Check sheet for the drawn part. Datum: minimum x, y, z corner. Units: mm. Round coordinates to 2 decimals unless told otherwise and drop trailing zeros. Order: outer loops, then holes, each group sorted by start corner. A loop starts at its lowest first (then second) coordinate and runs counter-clockwise, first axis right, second up. Notation, with made-up numbers: (48.5, 69) -> (77.5, 69) arc R16 cw to (77.5, 99) -> close; hole circle Ø10 at (-19, 65.5). An arc over 180 degrees is marked (long way). Use CSV: the item, a comma, the result in double quotes.
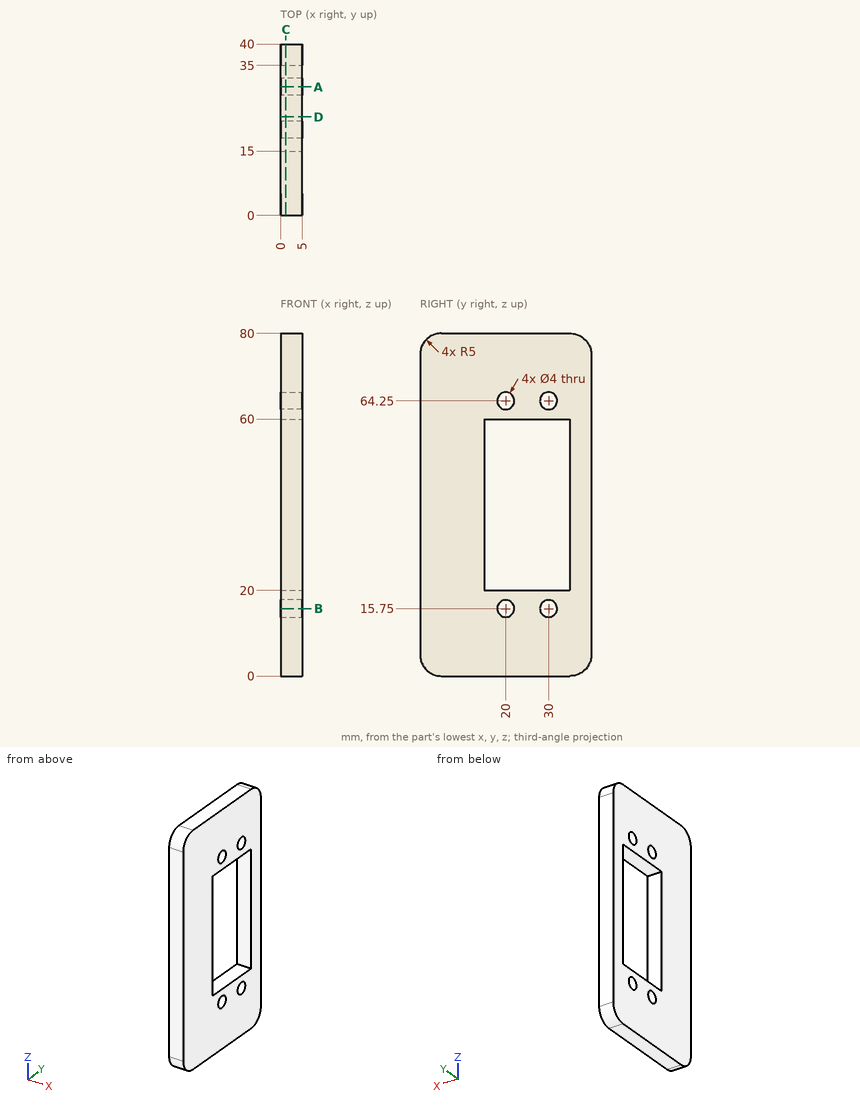
Q1. Sectioned sample at D-D, the plane y = 23. Enter the section's corners in (x, z).
Result sheet:
outline,"(0, 0) -> (5, 0) -> (5, 20) -> (0, 20) -> close; (0, 60) -> (5, 60) -> (5, 80) -> (0, 80) -> close"
Q2. Sectioned sample at C-C, the plane x = 1.2. Enter the section's corners in (y, z), then the cut area to 3 significant figures.
Result sheet:
outline,"(0, 5) arc R5 ccw to (5, 0) -> (35, 0) arc R5 ccw to (40, 5) -> (40, 75) arc R5 ccw to (35, 80) -> (5, 80) arc R5 ccw to (0, 75) -> close; hole (15, 20) -> (35, 20) -> (35, 60) -> (15, 60) -> close; hole circle Ø4 at (20, 15.75); hole circle Ø4 at (20, 64.25); hole circle Ø4 at (30, 15.75); hole circle Ø4 at (30, 64.25)"
area,"2,330 mm^2"
Q3. Go/stop test with a flat-tipped pin: pin 1 (3.5 mm diameter, centred on y = 20, z = 15.75, fed in from +X). Record where the tip stops, or that it passes through.
Result sheet:
pin 1,"passes through"
Q4. Scan lines: L1, parallel to Y at x = 1.35, z = 64.25; L2, parallel to Y at x = 1.6, z = 52.5; L3, parallel to Z at x = 2.35, y = 17. Record each from-to range of solid material in increasing order.
Result sheet:
L1,"y = 0 to 18, 22 to 28, 32 to 40"
L2,"y = 0 to 15, 35 to 40"
L3,"z = 0 to 20, 60 to 80"
Q5. Sectioned sample at A-A, the plane y = 30. Enter the section's corners in (x, z).
Result sheet:
outline,"(0, 0) -> (5, 0) -> (5, 13.75) -> (0, 13.75) -> close; (0, 17.75) -> (5, 17.75) -> (5, 20) -> (0, 20) -> close; (0, 60) -> (5, 60) -> (5, 62.25) -> (0, 62.25) -> close; (0, 66.25) -> (5, 66.25) -> (5, 80) -> (0, 80) -> close"
Q6. Sectioned sample at B-B, the plane z = 15.75. Enter the section's corners in (x, y), then the cut area to 3 significant figures.
Result sheet:
outline,"(0, 0) -> (5, 0) -> (5, 18) -> (0, 18) -> close; (0, 22) -> (5, 22) -> (5, 28) -> (0, 28) -> close; (0, 32) -> (5, 32) -> (5, 40) -> (0, 40) -> close"
area,"160 mm^2"
